The model under review builds one solid part; all positions refer to its coordinate system, in mm. Round coordinates to 2 decimals unless told otherwise and drop trailing zeros. Order: outer loops, then holes, each group sorted by start corner. A loop starts at its lowest first (then second) coordinate and runs counter-clockwise, first axis right, second up.
```python
from build123d import *

# Parameters (mm, degrees)
SKETCH1_W           = 280
SKETCH1_H           = 60
BOSS_EXTRUDE1_DEPTH = 10
SKETCH2_W           = 280
SKETCH2_H           = 10
BOSS_EXTRUDE2_DEPTH = 5
SKETCH3_R           = 2.5
CUT_EXTRUDE1_DEPTH  = 287.749019179
FILLET1_R           = 10
FILLET2_R           = 1
FILLET3_R           = 1
FILLET4_R           = 1


with BuildPart() as part:
    # Sketch1 → Boss-Extrude1 (new body)
    with BuildSketch(Plane(origin=(0, 0, 0), x_dir=(1, 0, 0), z_dir=(0, 1, 0))):
        with Locations((0, -30)):
            Rectangle(SKETCH1_W, SKETCH1_H)
    extrude(amount=BOSS_EXTRUDE1_DEPTH)

    # Sketch2 → Boss-Extrude2 (add)
    with BuildSketch(Plane(origin=(0, 10, 0), x_dir=(1, 0, 0), z_dir=(0, 1, 0))):
        with Locations((0, -55)):
            Rectangle(SKETCH2_W, SKETCH2_H)
    extrude(amount=BOSS_EXTRUDE2_DEPTH)

    # Sketch3 → Cut-Extrude1 (cut, through all)
    with BuildSketch(Plane(origin=(140, 0, 0), x_dir=(0, 0, -1), z_dir=(1, 0, 0))):
        with Locations((-55, 9.5)):
            Circle(SKETCH3_R)
    extrude(amount=-CUT_EXTRUDE1_DEPTH, mode=Mode.SUBTRACT)

    # Fillet1
    fillet1_edges = [part.edges().sort_by_distance(p)[0] for p in [
        (0, 0, 60),
    ]]
    fillet(fillet1_edges, radius=FILLET1_R)

    # Fillet2
    fillet2_edges = [part.edges().sort_by_distance(p)[0] for p in [
        (0, 15, 60),
    ]]
    fillet(fillet2_edges, radius=FILLET2_R)

    # Fillet3
    fillet3_edges = [part.edges().sort_by_distance(p)[0] for p in [
        (0, 15, 50),
    ]]
    fillet(fillet3_edges, radius=FILLET3_R)

    # Fillet4
    fillet4_edges = [part.edges().sort_by_distance(p)[0] for p in [
        (0, 10, 50),
    ]]
    fillet(fillet4_edges, radius=FILLET4_R)


solid = part.part
```
(1) To check wall thickness, follow probe 1 along Z at (x, y) = (-105, 9); probe 2 along Y at (x, z) = (105.5, 53); probe 3 along Y at (x, z) = (57, 5). State the ranges of each line that lie inside material, in increasing order.
Data:
probe 1: z = 0 to 52.55, 57.45 to 59.95
probe 2: y = 0.46 to 8, 11 to 15
probe 3: y = 0 to 10
(2) Consider section B-B (z = 55). Write out the cut boundary in (x, y).
Data:
outline: (-140, 1.34) - (140, 1.34) - (140, 7) - (-140, 7) - close; (-140, 12) - (140, 12) - (140, 15) - (-140, 15) - close
(3) Consider section A-A (x = -90). Write out the cut boundary in (y, z).
Data:
outline: (0, 0) - (10, 0) - (10, 49) arc R1 cw to (11, 50) - (14, 50) arc R1 ccw to (15, 51) - (15, 59) arc R1 ccw to (14, 60) - (10, 60) arc R10 ccw to (0, 50) - close; hole circle Ø5 at (9.5, 55)
(4) Insertion check: pin 1 (3.5 mm diameter, centred on x = 61.5, y = 12, fed in from -Z); pin 2 (5 mm diameter, centred on x = -85.5, z = 34, fed in from +Y); pin 3 (1 mm diameter, centred on x = -55.5, y = 6.5, fed in from +Z). Each pin has a flat end and moves straight along its axis. Give the tip position at first contact, or say it passes through.
Data:
pin 1: stops at z = 49.66
pin 2: stops at y = 10
pin 3: stops at z = 59.54
(5) Consider section D-D (z = 8.5). Write out the cut boundary in (x, y).
Data:
outline: (-140, 0) - (140, 0) - (140, 10) - (-140, 10) - close
(6) Draft analysis for pull direction Z (two halves, no side actions). For faces 1 (the flat face through (-2, 10, 24)), 2 (the flat face through (-2, 5, 0)), 3 (the cylindrical face through (1.96, 8.54, 52.69)), state which applies: pulls with the +Z half, pulls with the -Z half, needs draft (parallel to the pull), parting line crosses it, or undercut.
Data:
face 1: needs draft
face 2: pulls with the -Z half
face 3: undercut
(7) Consider section C-C (y = 2.5). Write out the cut boundary in (x, z).
Data:
outline: (-140, 0) - (140, 0) - (140, 56.61) - (-140, 56.61) - close
